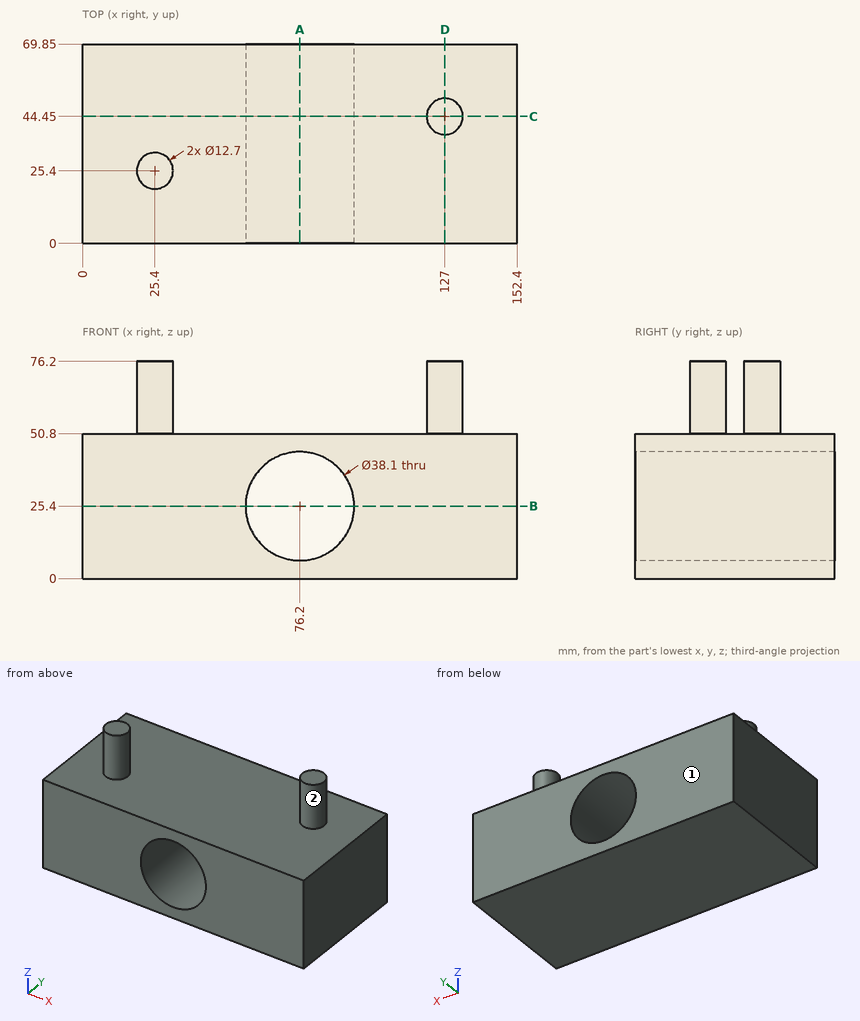
The figure shows three views and two pictorial views of one solid part (mm, origin at its lowest corner). Answer the questions. A direction names the side the tool comes from. Give positions to 0.01 mm unless a question says otherwise; leave off trailing zeros. Loops run counter-clockwise (first coordinate to the right, second up) from the corner with the lowest first, then second, coordinate; pieces in that order, holes last. Notation, with made-up numbers: (61.25, 18) - (75.25, 18) arc R14 cw to (75.25, 35) - close; hole circle Ø3 at (50, 11). An arc over 180 degrees is marked (long way). Answer in a Markdown table with one row per item.
(1) A tool of negligible diameter and unlimited length cuts with its end or side. For the marked faces 1 and 2, from which of +Z, -Z, +X, -X, +Y, -Y can it reach the whole face along a straight path? Write none if from no direction.
Results list:
| item | result |
|---|---|
| face 1 | +Z, -Z, +X, -X, +Y |
| face 2 | +Z |
(2) Section D-D (x = 127) is taken. Give the vertices of the cut face in (y, z), and give its area (3 significant figures).
Results list:
| item | result |
|---|---|
| outline | (0, 0) - (69.85, 0) - (69.85, 50.8) - (50.8, 50.8) - (50.8, 76.2) - (38.1, 76.2) - (38.1, 50.8) - (0, 50.8) - close |
| area | 3,870 mm² |
(3) Consider L1, parallel to Z at x = 76.2, y = 55; L2, parallel to X at y = 50, z = 25; L3, parallel to Z at x = 63.5, y = 27.5. Determine where each line is inside the solid, lowest interval first. Write a range as [from, to].
Results list:
| item | result |
|---|---|
| L1 | z = [0, 6.35], [44.45, 50.8] |
| L2 | x = [0, 57.15], [95.25, 152.4] |
| L3 | z = [0, 11.2], [39.6, 50.8] |
(4) Flat-ended cylindrical pins translate along their axes: pin 1 Ø2 at (y, z) = (36.5, 67.5) entering from +X; pin 2 Ø12 at (y, z) = (24, 66) entering from -X; pin 3 Ø3 at (x, z) = (22, 54) entering from -Y. Find the tip coordinate at first contact, or state that the pin passes through.
Results list:
| item | result |
|---|---|
| pin 1 | passes through |
| pin 2 | stops at x = 19.05 |
| pin 3 | stops at y = 19.34 |
(5) Section B-B (z = 25.4) is taken. Give the vertices of the cut face in (x, y), and give its area (3 significant figures).
Results list:
| item | result |
|---|---|
| outline | (0, 0) - (57.15, 0) - (57.15, 69.85) - (0, 69.85) - close; (95.25, 0) - (152.4, 0) - (152.4, 69.85) - (95.25, 69.85) - close |
| area | 7,980 mm² |
(6) Section C-C (y = 44.45) is taken. Give the vertices of the cut face in (x, z), and give its area (3 significant figures).
Results list:
| item | result |
|---|---|
| outline | (0, 0) - (152.4, 0) - (152.4, 50.8) - (133.35, 50.8) - (133.35, 76.2) - (120.65, 76.2) - (120.65, 50.8) - (0, 50.8) - close; hole circle Ø38.1 at (76.2, 25.4) |
| area | 6,920 mm² |
(7) Section A-A (x = 76.2) is taken. Give the vertices of the cut face in (y, z).
Results list:
| item | result |
|---|---|
| outline | (0, 0) - (69.85, 0) - (69.85, 6.35) - (0, 6.35) - close; (0, 44.45) - (69.85, 44.45) - (69.85, 50.8) - (0, 50.8) - close |
